Verification items for this drawing (mm, ordinates from the low corner). A direction names the side the tool comes from. Coordinates: 2 decimals unless noted, no trailing zeros. Loops run counter-clockwise (first coordinate to the right, second up) from the corner with the lowest first, then second, coordinate; pieces in that order, holes last.
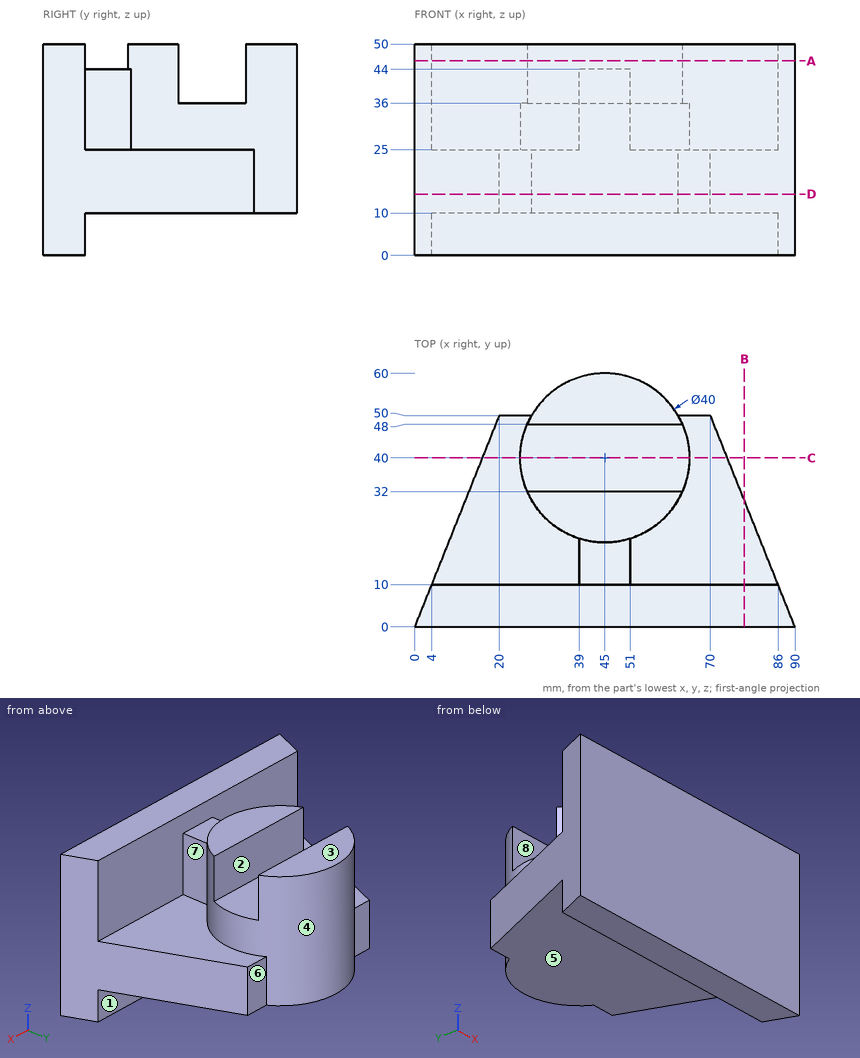
(1) Draft check along Y on the marked faces 1, 2 and 3. Enter one of: pulls with the +Y half, pulls with the -Y half, needs draft (parallel to the pull), parting line crosses it, or undercut.
(2) Section check B-B, the plane x = 78. Enter the section's corners in (y, z).
(3) Scan lines: line 1 along Y through (x, z) = (28, 47); line 2 along Y through (x, z) = (30.5, 26); line 3 along Y through (x, z) = (10.5, 45.5). Record each from-to range of solid material in increasing order.
(4) Section check A-A, the plane z = 46. Enter the section's corners in (x, y), plus the area to 3 significant figures.
(5) Section check D-D, the plane z = 14.5. Enter the section's corners in (x, y).
(6) Gauge pin test, flat ends, axial feed: P1, Ø5, axis at x = 18, z = 16.5, coming from the +Y side; P2, Ø1, axis at x = 30, y = 33.5, coming from the +Z side; P3, Ø7, axis at x = 38.5, z = 45.5, coming from the +Y side. Record the tip position at first contact, or that the pin passes through.
(7) Set-up check for the marked faces 4, 5, 6, 7 and 8: record each of +Z, -Z, +X, -X, +Y, -Y from which the full face is reachable in a straight line by a thin tool's end or side.
(8) Section check C-C, the plane y = 40. Enter the section's corners in (x, z), plus the area to 3 significant figures.
Determined:
1. face 1: pulls with the +Y half
1. face 2: undercut
1. face 3: needs draft
2. outline: (0, 0) - (10, 0) - (10, 10) - (30, 10) - (30, 25) - (10, 25) - (10, 50) - (0, 50) - close
3. line 1: y = 0 to 10, 29.46 to 32, 48 to 50.54
3. line 2: y = 0 to 10, 26.23 to 53.77
3. line 3: y = 0 to 10
4. outline: (0, 0) - (90, 0) - (86, 10) - (4, 10) - close; (26.67, 32) arc R20 ccw to (63.33, 32) - close; (26.67, 48) - (63.33, 48) arc R20 ccw to start
4. area: 1,490 mm2
5. outline: (0, 0) - (90, 0) - (70, 50) - (62.32, 50) arc R20 ccw to (27.68, 50) - (20, 50) - close
6. P1: stops at y = 50
6. P2: stops at z = 36
6. P3: stops at y = 59.77
7. face 4: +Z
7. face 5: -Z, +X, -X, +Y
7. face 6: +Z, -Z, +X, +Y
7. face 7: +Z, +X
7. face 8: +Z, +X, -X
8. outline: (16, 10) - (74, 10) - (74, 25) - (65, 25) - (65, 36) - (25, 36) - (25, 25) - (16, 25) - close
8. area: 1,310 mm2
